```python
from build123d import *

# Parameters (mm, degrees)
RESSALTO_EXTRUS_O1_DEPTH      = 4
FURO_COM_FOLGA_DE_M2_51_D     = 2.9
FURO_COM_FOLGA_DE_M2_51_DEPTH = 7.25
FURO_COM_FOLGA_DE_M2_51_TIP   = 0.871247898
FUROS_GUIA_COM_8_0MM1_D       = 8
FUROS_GUIA_COM_8_0MM1_DEPTH   = 7.25
FUROS_GUIA_COM_8_0MM1_TIP     = 2.403442476


with BuildPart() as part:
    # Esboço1 → Ressalto-extrusão1 (new body)
    with BuildSketch(Plane.XY):
        with BuildLine():
            Line((-40, 75), (40, 75))
            ThreePointArc((40, 75), (0, -85), (-40, 75))
        make_face()
    extrude(amount=RESSALTO_EXTRUS_O1_DEPTH)

    # Furo com folga de M2.51
    with Locations(Plane(origin=(-53.033008589, 53.033008589, 4), x_dir=(1, 0, 0), z_dir=(0, 0, 1))):
        with Locations((0, 0), (106.066017178, 0), (101.242079315, -110.486341823), (4.823937863, -110.486341823)):
            Hole(FURO_COM_FOLGA_DE_M2_51_D / 2, depth=FURO_COM_FOLGA_DE_M2_51_DEPTH)
            with Locations((0, 0, -(FURO_COM_FOLGA_DE_M2_51_DEPTH + FURO_COM_FOLGA_DE_M2_51_TIP / 2))):  # 118° drill point
                Cone(0, FURO_COM_FOLGA_DE_M2_51_D / 2, FURO_COM_FOLGA_DE_M2_51_TIP, mode=Mode.SUBTRACT)

    # Furos-guia com Ø8.0mm1
    with Locations(Plane(origin=(-64.951905284, 37.5, 4), x_dir=(1, 0, 0), z_dir=(0, 0, 1))):
        with Locations((0, 0), (0, -75), (129.903810568, 0), (129.903810568, -75)):
            Hole(FUROS_GUIA_COM_8_0MM1_D / 2, depth=FUROS_GUIA_COM_8_0MM1_DEPTH)
            with Locations((0, 0, -(FUROS_GUIA_COM_8_0MM1_DEPTH + FUROS_GUIA_COM_8_0MM1_TIP / 2))):  # 118° drill point
                Cone(0, FUROS_GUIA_COM_8_0MM1_D / 2, FUROS_GUIA_COM_8_0MM1_TIP, mode=Mode.SUBTRACT)


solid = part.part
```
Input: part model. Units: mm. Frame: model coordinates. Coordinates: 2 decimals unless noted, no trailing zeros. Write each loop counter-clockwise with the first axis right and the second up, starting at its lowest first coordinate (ties: lowest second). Pieces come first, ordered by that corner, then holes. Notation, with made-up numbers: M 54,15 L 77,15 A16 ccw 77,42 Z; hole C -10.5,13.5 d2. An arc over 180 degrees is marked long. Use one line per item in the form item = value.
Q1. Draft query along Y for faces 1 (the face through (3.15, -84.94, 1.97)), 2 (the face through (62.8, 40.87, 1.97)), 3 (the face through (1, -4, 4)). Return one class per face: released by +Y, released by -Y, zero draft, split by the parting line, or undercut.
Answer below:
face_1 = split by the parting line
face_2 = undercut
face_3 = zero draft
Q2. First-contact query: pin 1 (5 mm diameter, centred on x = -64.95, y = 37.5, fed in from +Z); pin 2 (1.5 mm diameter, centred on x = -63.5, z = 3.5, fed in from +Y); pin 3 (9 mm diameter, centred on x = 64.95, y = 37.5, fed in from +Z). Flat tips, straight axial feed; report the tip coordinate or a pass-through.
Answer below:
pin_1 = through
pin_2 = 57.34
pin_3 = 4
Q3. Section D-D (y = -18.5). Return loops of the section in (x, z).
Answer below:
outline = M -82.96,0 L 82.96,0 L 82.96,4 L -82.96,4 Z
Q4. Material intervals for probe 1 along Y at (x, z) = (-48, 0.3); probe 2 along X at (y, z) = (-62, 3.45); probe 3 along X at (y, z) = (-5, 1.1), sorted ascending. Write a range as from..to.
Answer below:
probe_1 = -70.15..-58.89, -56.02..70.15
probe_2 = -58.15..58.15
probe_3 = -84.85..84.85
Q5. Section B-B (y = 37.5). Return loops of the section in (x, z), plus the area to 3 significant figures.
Answer below:
outline = M -76.28,0 L -68.95,0 L -68.95,4 L -76.28,4 Z; M -60.95,0 L 60.95,0 L 60.95,4 L -60.95,4 Z; M 68.95,0 L 76.28,0 L 76.28,4 L 68.95,4 Z
area = 546 mm²
Q6. Section C-C (x = -57.5). Return loops of the section in (y, z).
Answer below:
outline = M -62.6,0 L 62.6,0 L 62.6,4 L -62.6,4 Z
Q7. Section A-A (z = 3.3). Count the separate pieces of the cut face and the enclosed holes in it, plus the area to 3 significant figures.
Answer below:
separate_pieces = 1
enclosed_holes = 8
area = 21,900 mm²
